Geometry: final body of the model. Coordinates: model frame, mm. Give positions to 0.01 mm unless a question says otherwise; leave off trailing zeros. Order: outer loops, then holes, each group sorted by start corner. A loop starts at its lowest first (then second) coordinate and runs counter-clockwise, first axis right, second up. Notation, with made-up numbers: (55, 46.25) -> (79, 46.25) arc R18 cw to (79, 62.25) -> close; hole circle Ø7 at (14.5, 16.25). An arc over 180 degrees is marked (long way). Write item = value, one per line.
```python
from build123d import *

# Parameters (mm, degrees)
BOSS_EXTRUDE1_DEPTH = 5


with BuildPart() as part:
    # Sketch1 → Boss-Extrude1 (new body)
    with BuildSketch(Plane.XY):
        with BuildLine():
            Line((-41.5, -38), (-41.5, 80))
            Line((-41.5, 80), (27.40518995, 80))
            ThreePointArc((27.40518995, 80), (35.56101739, 75.786404649), (36.843773513, 66.696495753))
            Line((36.843773513, 66.696495753), (13.5, 0))
            Line((13.5, 0), (-41.5, -38))
        make_face()
    extrude(amount=BOSS_EXTRUDE1_DEPTH)


solid = part.part
```
1) Section query B-B (x = -29.5). Output: boundary loops of the cut face in (y, z), plus the area to 3 significant figures.
Check sheet entries:
outline = (-29.71, 0) -> (80, 0) -> (80, 5) -> (-29.71, 5) -> close
area = 549 mm²
2) Section query A-A (z = 4.25). Output: boundary loops of the cut face in (x, y), plus the area to 3 significant figures.
Check sheet entries:
outline = (-41.5, -38) -> (13.5, 0) -> (36.84, 66.7) arc R10 ccw to (27.41, 80) -> (-41.5, 80) -> close
area = 6,520 mm²
3) First-contact query: P1, Ø2, axis at x = -27.5, z = 4.5, coming from the -Y side; P2, Ø3, axis at y = 27.5, z = 2, coming from the +X side. Flat tips, straight axial feed; report the tip coordinate or a pass-through.
Check sheet entries:
P1 = -29.02
P2 = 23.65
4) Line query: line 1 (X direction, y = 54, z = 3.85); line 2 (Y direction, x = -21, z = 1.5); line 3 (X direction, y = -0.5, z = 4.8). Output: solid intervals per line, ascending. Write a range as from..to.
Check sheet entries:
line_1 = -41.5..32.4
line_2 = -23.84..80
line_3 = -41.5..12.78
5) Section query C-C (y = 55). Output: boundary loops of the cut face in (x, z), plus the area to 3 significant figures.
Check sheet entries:
outline = (-41.5, 0) -> (32.75, 0) -> (32.75, 5) -> (-41.5, 5) -> close
area = 371 mm²
